```python
from build123d import *

# Parameters (mm, degrees)
F0_R     = 100
F0_R_2   = 90
F1_DEPTH = 20
F2_DEPTH = 320
F3_R     = 55
F4_DEPTH = 147
F5_R     = 10


with BuildPart() as f1:
    # F0 (on Top) → F1 (new body)
    with BuildSketch(Plane.XY):
        Circle(F0_R)
        Circle(F0_R_2, mode=Mode.SUBTRACT)
    extrude(amount=F1_DEPTH)

    # F0 (on Top) → F2 (join)
    with BuildSketch(Plane.XY):
        Circle(F0_R_2)
    extrude(amount=F2_DEPTH)

    # F3 (on Front) → F4 (cut, symmetric)
    with BuildSketch(Plane.XZ):
        with Locations((0, 170)):
            Circle(F3_R)
    extrude(amount=F4_DEPTH, both=True, mode=Mode.SUBTRACT)

    # F5
    f5_edges = [f1.edges().sort_by_distance(p)[0] for p in [
        (-100, 0, 0),
    ]]
    fillet(f5_edges, radius=F5_R)


solid = f1.part
```
Check sheet for the modelled part. Datum: model origin and axes. Units: mm. A direction names the side the tool comes from. Round coordinates to 2 decimals unless told otherwise and drop trailing zeros. Write each loop counter-clockwise with the first axis right and the second up, starting at its lowest first coordinate (ties: lowest second). Pieces come first, ordered by that corner, then holes. Notation, with made-up numbers: (29.25, -38.5) -> (66.25, -38.5) arc R35 cw to (66.25, 0.5) -> close; hole circle Ø3 at (-20.5, 89). An arc over 180 degrees is marked (long way). Put each result on its own line as item: value.
(1) Material ranges on line 1 (Z direction, x = 0, y = 23.5); line 2 (X direction, y = 27.5, z = 170); line 3 (Z direction, x = 13, y = 82.5), recorded low to high.
Values found:
line 1: z = 0 to 115, 225 to 320
line 2: x = -85.7 to -55, 55 to 85.7
line 3: z = 0 to 116.56, 223.44 to 320
(2) Mould release check, pull along X, two halves, no side actions. Record for faces 1 (the face through (95.38, 30.04, 14.93)), 2 (the face through (-1, 1, 320)), 3 (the face through (29.568, -1.26, 216.376)): released by +X, released by -X, zero draft, split by the parting line, or undercut.
Values found:
face 1: split by the parting line
face 2: zero draft
face 3: undercut
(3) Sectioned sample at B-B (y = 0). Enter the section's corners in (x, z), plus the area to 3 significant figures.
Values found:
outline: (-100, 10) arc R10 ccw to (-90, 0) -> (90, 0) arc R10 ccw to (100, 10) -> (100, 20) -> (90, 20) -> (90, 320) -> (-90, 320) -> (-90, 20) -> (-100, 20) -> close; hole circle Ø110 at (0, 170)
area: 48,500 mm^2
(4) Go/stop test with flat-tipped pins: pin 1 Ø8 at (y, z) = (11, 177.5) entering from -X; pin 2 Ø5 at (x, z) = (51, 86) entering from -Y; pin 3 Ø3 at (y, z) = (-16, 280.5) entering from +X. Record where each tip stops, or that it passes through.
Values found:
pin 1: stops at x = -89.73
pin 2: stops at y = -75.81
pin 3: stops at x = 88.82
(5) Sectioned sample at A-A (x = 0). Enter the section's corners in (y, z).
Values found:
outline: (-100, 10) arc R10 ccw to (-90, 0) -> (90, 0) arc R10 ccw to (100, 10) -> (100, 20) -> (90, 20) -> (90, 115) -> (-90, 115) -> (-90, 20) -> (-100, 20) -> close; (-90, 225) -> (90, 225) -> (90, 320) -> (-90, 320) -> close
(6) Tool access check on faces 4 (the face through (-1, 1, 0)), 5 (the face through (-82, 38, 20)). Record the directions out of +Z, -Z, +X, -X, +Y, -Y that give a thin tool (end or side, any length) a straight path to the whole face; none if there is none.
Values found:
face 4: -Z, +X, -X, +Y, -Y
face 5: +Z
(7) Sectioned sample at D-D (z = 251.5). Enter the section's corners in (x, y).
Values found:
outline: circle Ø180 at (0, 0)
(8) Sectioned sample at C-C (z = 170). Enter the section's corners in (x, y).
Values found:
outline: (-55, -71.24) -> (-55, 71.24) arc R90 ccw to start; (55, -71.24) arc R90 ccw to (55, 71.24) -> close
